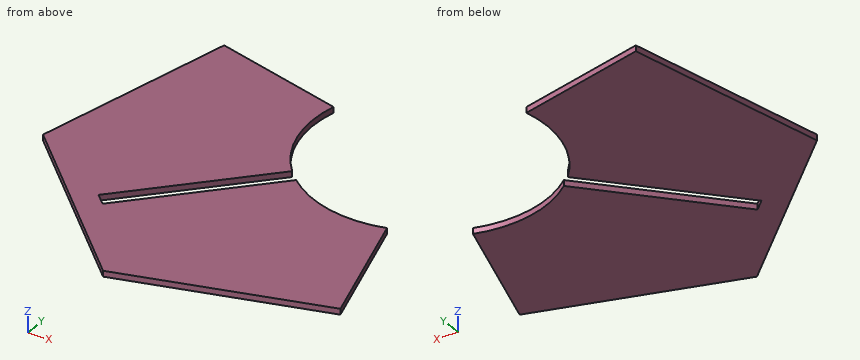
from build123d import *

# Parameters (mm, degrees)
BOSS_EXTRU_1_DEPTH      = 4
ENL_V_MAT_EXTRU_2_DEPTH = 10


with BuildPart() as part:
    # Esquisse1 → Boss.-Extru.1 (new body)
    with BuildSketch(Plane.XY):
        with BuildLine():
            Line((-252.479191453, -50.401668407), (-36.99219102, -254.789419126))
            Line((-36.99219102, -254.789419126), (48.52273895, -164.630612218))
            Line((48.52273895, -164.630612218), (22.191553545, -75.81909358))
            ThreePointArc((22.191553545, -75.81909358), (-16.163403148, -77.442245684), (-50.738038063, -60.758962249))
            Line((-50.738038063, -60.758962249), (-129.87807622, -144.196689689))
            Line((-129.87807622, -144.196689689), (-137.13353078, -137.314947241))
            Line((-137.13353078, -137.314947241), (-57.993492623, -53.8772198))
            ThreePointArc((-57.993492623, -53.8772198), (-76.480137606, -20.232290272), (-76.885637492, 18.154854653))
            Line((-76.885637492, 18.154854653), (-166.964261484, 39.757138501))
            Line((-166.964261484, 39.757138501), (-252.479191453, -50.401668407))
        make_face()
    extrude(amount=-BOSS_EXTRU_1_DEPTH)

    # Esquisse3 → Enlèv. mat.-Extru.2 (cut)
    with BuildSketch(Plane.XY):
        Polygon((-166.964261484, 39.757138501), (-200.425980015, -99.773736244), (-252.479191453, -50.401668407), align=None)
        Polygon((-36.99219102, -254.789419126), (48.52273895, -164.630612218), (-89.045402457, -205.417351289), align=None)
    extrude(amount=-ENL_V_MAT_EXTRU_2_DEPTH, mode=Mode.SUBTRACT)


solid = part.part
Geometry: final body of the model. Coordinates: model frame, mm. Coordinates: 2 decimals unless noted, no trailing zeros. Order: outer loops, then holes, each group sorted by start corner. A loop starts at its lowest first (then second) coordinate and runs counter-clockwise, first axis right, second up.
1) Ray query, probe 1 along Y at (x, z) = (-96.5, -0.3); probe 2 along X at (y, z) = (-86, -1.3); probe 3 along Y at (x, z) = (-73, -1.8). Return the intervals inside material, ascending.
Result sheet:
probe 1: y = -198.35 to -109.01, -94.47 to 22.86
probe 2: x = -197.12 to -88.46, -74.68 to 25.21
probe 3: y = -200.66 to -84.23, -69.7 to -30.54
2) Section A-A (x = -114.5). Return loops of the section in (y, z), then the cut area to 3 significant figures.
Result sheet:
outline: (-181.27, -4) - (-127.98, -4) - (-127.98, 0) - (-181.27, 0) - close; (-113.45, -4) - (27.18, -4) - (27.18, 0) - (-113.45, 0) - close
area: 776 mm2
3) Section D-D (y = -23.5). Return loops of the section in (x, z), then the cut area to 3 significant figures.
Result sheet:
outline: (-182.13, -4) - (-75.55, -4) - (-75.55, 0) - (-182.13, 0) - close
area: 426 mm2
4) Section B-B (y = -117). Return loops of the section in (x, z), then the cut area to 3 significant figures.
Result sheet:
outline: (-182.26, -4) - (-117.86, -4) - (-117.86, 0) - (-182.26, 0) - close; (-104.08, -4) - (34.4, -4) - (34.4, 0) - (-104.08, 0) - close
area: 812 mm2
5) First-contact query: P1, Ø1.5, axis at y = -17.5, z = -1.5, coming from the +X side. Flat tip, straight axial feed; report the tip coordinate or a pass-through.
Result sheet:
P1: stops at x = -76.97
6) Section C-C (z = -2.2). Return loops of the section in (x, y).
Result sheet:
outline: (-200.43, -99.77) - (-89.05, -205.42) - (48.52, -164.63) - (22.19, -75.82) arc R78.84 cw to (-50.74, -60.76) - (-129.88, -144.2) - (-137.13, -137.31) - (-57.99, -53.88) arc R78.84 cw to (-76.89, 18.15) - (-166.96, 39.76) - close
